```python
from build123d import *

# Parameters (mm, degrees)
F0_W     = 4.1
F0_H     = 2.55
F0_W_2   = 3.1
F0_H_2   = 1.55
F1_DEPTH = 38.1
F0_R     = 9.525
F2_DEPTH = 6.35
F3_W     = 4.1
F3_H     = 2.55
F3_W_2   = 3.1
F3_H_2   = 1.55
F4_DEPTH = 1


with BuildPart() as f1:
    # F0 (on Front) → F1 (new body)
    with BuildSketch(Plane.XZ):
        Rectangle(F0_W, F0_H)
        Rectangle(F0_W_2, F0_H_2, mode=Mode.SUBTRACT)
    extrude(amount=F1_DEPTH)

    # F0 (on Front) → F2 (join)
    with BuildSketch(Plane.XZ):
        Circle(F0_R)
        Rectangle(F0_W, F0_H, mode=Mode.SUBTRACT)
    extrude(amount=F2_DEPTH)

    # F3 (on face) → F4 (join)
    with BuildSketch(Plane.XZ.offset(38.1)):
        Rectangle(F3_W, F3_H)
        Rectangle(F3_W_2, F3_H_2, mode=Mode.SUBTRACT)
        Rectangle(F3_W_2, F3_H_2)
    extrude(amount=-F4_DEPTH)


solid = f1.part
```
Model file for the job. Use its own axes, mm. A direction names the side the tool comes from. Round coordinates to 2 decimals unless told otherwise and drop trailing zeros. Write each loop counter-clockwise with the first axis right and the second up, starting at its lowest first coordinate (ties: lowest second). Pieces come first, ordered by that corner, then holes. Notation, with made-up numbers: (87.25, -22) - (97.25, -22) arc R20 cw to (97.25, -1) - close; hole circle Ø5 at (-10.5, 19). An arc over 180 degrees is marked (long way). One line per item, written item: value.
(1) 3-axis set-ups, long thin cutter, end or side, ignore diameter. For faces 5 (the flat face through (-1.55, -18, 0)), 6 (the flat face through (0, -22, -1.275)), 7 (the flat face through (-2.05, -22, 0)): which of +Z, -Z, +X, -X, +Y, -Y reach the whole face in a straight line?
Values follow:
face 5: +Y
face 6: -Z, +X, -X, -Y
face 7: +Z, -Z, -X, -Y
(2) Cut at C-C, the plane x = 0. Give the cut face in (y, z) (3 decimals).
Values follow:
outline: (-38.1, -1.275) - (-6.35, -1.275) - (-6.35, -9.525) - (0, -9.525) - (0, -0.775) - (-37.1, -0.775) - (-37.1, 0.775) - (0, 0.775) - (0, 9.525) - (-6.35, 9.525) - (-6.35, 1.275) - (-38.1, 1.275) - close
(3) Drop flat-ended pins along their axis: P1, Ø10, axis at x = 6.5, z = 5.5, coming from the -Y side; P2, Ø1.2, axis at y = -25.5, z = -0.5, coming from the -X side; P3, Ø1.2, axis at x = 0, y = -28, coming from the -Z side (3 decimals). Give the stop position or say it passes through.
Values follow:
P1: stops at y = -6.35
P2: stops at x = -2.05
P3: stops at z = -1.275
(4) Cut at B-B, the plane z = 0. Give the cut face in (x, y) (3 decimals), plus the area to 3 significant figures.
Values follow:
outline: (-9.525, -6.35) - (-2.05, -6.35) - (-2.05, -38.1) - (2.05, -38.1) - (2.05, -6.35) - (9.525, -6.35) - (9.525, 0) - (1.55, 0) - (1.55, -37.1) - (-1.55, -37.1) - (-1.55, 0) - (-9.525, 0) - close
area: 136 mm²
(5) Wall check: probe 1 along Z at (x, y) = (-0.75, -8) (3 decimals); probe 2 along X at (y, z) = (-32, 0.25); probe 3 along Y at (x, z) = (0.5, -7.75). Give the ranges that are in metal, low to high.
Values follow:
probe 1: z = -1.275 to -0.775, 0.775 to 1.275
probe 2: x = -2.05 to -1.55, 1.55 to 2.05
probe 3: y = -6.35 to 0
(6) Cut at A-A, the plane y = -4.5. Give the cut face in (x, z) (3 decimals), plus the area to 3 significant figures.
Values follow:
outline: circle Ø19.05 at (0, 0); hole (-1.55, -0.775) - (1.55, -0.775) - (1.55, 0.775) - (-1.55, 0.775) - close
area: 280 mm²
(7) Cut at D-D, the plane y = -16.5. Give the cut face in (x, z) (3 decimals).
Values follow:
outline: (-2.05, -1.275) - (2.05, -1.275) - (2.05, 1.275) - (-2.05, 1.275) - close; hole (-1.55, -0.775) - (1.55, -0.775) - (1.55, 0.775) - (-1.55, 0.775) - close
(8) Two-plate mould, pull along X, no slides. Class faces 1 (the flat face through (0, -18, -0.775)), 2 (the flat face through (0, -18, 0.775)), 3 (the flat face through (0, -22, 1.275)), 4 (the flat face through (2.05, -22, 0)): pulls with the +X half, pulls with the -X half, needs draft (parallel to the pull), parting line crosses it, or undercut.
Values follow:
face 1: undercut
face 2: undercut
face 3: needs draft
face 4: pulls with the +X half
